Model file for the job. Use its own axes, mm. A direction names the side the tool comes from. Coordinates: 2 decimals unless noted, no trailing zeros. Loops run counter-clockwise (first coordinate to the right, second up) from the corner with the lowest first, then second, coordinate; pieces in that order, holes last.
from build123d import *

# Parameters (mm, degrees)
SKETCH_1_W          = 112
SKETCH_1_H          = 70
EXTRUDE_1_DEPTH     = 126
SKETCH_2_W          = 110
SKETCH_2_H          = 69
CUT_EXTRUDE_1_DEPTH = 125
SKETCH_3_W          = 112
SKETCH_3_H          = 1
EXTRUDE_2_DEPTH     = 12
SKETCH_4_W          = 22
SKETCH_4_H          = 1
EXTRUDE_3_DEPTH     = 12
CUT_EXTRUDE_2_DEPTH = 10
SKETCH_6_R          = 2.75
CUT_EXTRUDE_3_DEPTH = 190.770914526
CUT_EXTRUDE_5_REACH = 192.137
SKETCH_8_W          = 17
SKETCH_8_H          = 24
SKETCH_9_R          = 2.5
CUT_EXTRUDE_6_DEPTH = 10


with BuildPart() as part:
    # 草图1 → 拉伸1 (new body)
    with BuildSketch(Plane.XY):
        with Locations((56, 35)):
            Rectangle(SKETCH_1_W, SKETCH_1_H)
    extrude(amount=EXTRUDE_1_DEPTH)

    # 草图2 → 切除-拉伸1 (cut)
    with BuildSketch(Plane.XY.offset(126)):
        with Locations((56, 35.5)):
            Rectangle(SKETCH_2_W, SKETCH_2_H)
    extrude(amount=-CUT_EXTRUDE_1_DEPTH, mode=Mode.SUBTRACT)

    # 草图3 → 拉伸2 (add)
    with BuildSketch(Plane(origin=(0, 0, 0), x_dir=(-1, 0, 0), z_dir=(0, 0, -1))):
        with Locations((-56, 69.5)):
            Rectangle(SKETCH_3_W, SKETCH_3_H)
    extrude(amount=EXTRUDE_2_DEPTH)

    # 草图4 → 拉伸3 (add)
    with BuildSketch(Plane(origin=(112, 0, 0), x_dir=(0, 0, -1), z_dir=(1, 0, 0))):
        with Locations((-86, 69.5)):
            Rectangle(SKETCH_4_W, SKETCH_4_H)
    extrude_3 = extrude(amount=EXTRUDE_3_DEPTH)

    # 草图5 → 切除-拉伸2 (cut)
    with BuildSketch(Plane(origin=(0, 70, 0), x_dir=(-1, 0, 0), z_dir=(0, 1, 0))):
        Polygon((-112, 75), (-124, 87), (-124, 75), align=None)
    cut_extrude_2 = extrude(amount=-CUT_EXTRUDE_2_DEPTH, mode=Mode.SUBTRACT)

    # 镜向1: 拉伸3 across plane
    add(extrude_3.mirror(Plane.ZY.offset(-56)))

    # 镜向2: 切除-拉伸2 across plane
    add(cut_extrude_2.mirror(Plane.ZY.offset(-56)), mode=Mode.SUBTRACT)

    # 草图6 → 切除-拉伸3 (cut, through all)
    with BuildSketch(Plane.XZ.offset(-69)):
        with Locations(Location((-6, 90, 0), (0, 0, 270))):
            Circle(SKETCH_6_R)
        with Locations(Location((118, 90, 0), (0, 0, 270))):
            Circle(SKETCH_6_R)
        with Locations(Location((16, -6, 0), (0, 0, 270))):
            Circle(SKETCH_6_R)
        with Locations(Location((96, -6, 0), (0, 0, 270))):
            Circle(SKETCH_6_R)
    extrude(amount=-CUT_EXTRUDE_3_DEPTH, mode=Mode.SUBTRACT)

    # 草图8 → 切除-拉伸5 (cut, up to next)
    with BuildSketch(Plane.ZY, mode=Mode.PRIVATE) as cut_extrude_5_sk1:
        with Locations((117.5, 20)):
            Rectangle(SKETCH_8_W, SKETCH_8_H)
    cut_extrude_5_tool1 = extrude(cut_extrude_5_sk1.sketch, amount=-CUT_EXTRUDE_5_REACH, mode=Mode.PRIVATE) & part.part
    add(cut_extrude_5_tool1.solids().sort_by_distance((0, 20, 117.5))[0], mode=Mode.SUBTRACT)

    # 草图9 → 切除-拉伸6 (cut)
    with BuildSketch(Plane.ZY):
        with Locations((20, 65)):
            Circle(SKETCH_9_R)
        with Locations((20, 55)):
            Circle(SKETCH_9_R)
        with Locations((50, 65)):
            Circle(SKETCH_9_R)
        with Locations((50, 55)):
            Circle(SKETCH_9_R)
        with Locations((76, 25)):
            Circle(SKETCH_9_R)
        with Locations((76, 15)):
            Circle(SKETCH_9_R)
    extrude(amount=-CUT_EXTRUDE_6_DEPTH, mode=Mode.SUBTRACT)


solid = part.part
Q1. Flat gauge pins, fed straight in: P1, Ø12, axis at y = 13, z = 6.5, coming from the +X side; P2, Ø3.5, axis at x = 64, z = -7, coming from the -Y side; P3, Ø1.5, axis at x = 110, y = 31, coming from the -Z side. Where does each tip first touch, or does it go through?
Answers:
P1: stops at x = 112
P2: stops at y = 69
P3: stops at z = 0
Q2. Drill centre lines: line 1 (Y direction, x = 0.6, z = 76); line 2 (X direction, y = 20, z = 78); line 3 (Z direction, x = 61.5, y = 48.5). Where is each one in solid material? Low to high.
Answers:
line 1: y = 0 to 12.5, 17.5 to 22.5, 27.5 to 70
line 2: x = 0 to 1, 111 to 112
line 3: z = 0 to 1
Q3. Slice it at B-B (z = 50). List the corners of the cut face in (x, y), and give its area (3 significant figures).
Answers:
outline: (0, 0) - (112, 0) - (112, 70) - (111, 70) - (111, 1) - (1, 1) - (1, 52.5) - (0, 52.5) - close; (0, 57.5) - (1, 57.5) - (1, 62.5) - (0, 62.5) - close; (0, 67.5) - (1, 67.5) - (1, 70) - (0, 70) - close
area: 240 mm2
Q4. Which spindle directions (+Z, -Z, +X, -X, +Y, -Y) get a long thin tool onto all of the face, cutting with end or side? Do faces 1 (the cylindrical face through (116.327, 69.493, 92.182)), 2 (the flat face through (-3, 69, 89)), 3 (the flat face through (111, 35, 64)), 4 (the flat face through (55, 0, 62)), 5 (the cylindrical face through (0.49, 54.04, 52.31)). Say none if no direction does.
Answers:
face 1: +Y, -Y
face 2: +Z, -Z, -X, -Y
face 3: +Z, +Y
face 4: +Z, -Z, +X, -X, -Y
face 5: -X
Q5. Mould opens along X. For faces 6 (the flat face through (1, 35, 64)), 7 (the flat face through (115, 69, 89)) say: +X half, -X half, draft (parallel to the pull), parting line (faces both ways), or undercut.
Answers:
face 6: undercut
face 7: draft
Q6. Slice it at C-C (x = 96). List the corners of the cut face in (y, z), and give its area (4 significant figures).
Answers:
outline: (0, 0) - (69, 0) - (69, -3.25) - (70, -3.25) - (70, 1) - (1, 1) - (1, 126) - (0, 126) - close; (69, -12) - (70, -12) - (70, -8.75) - (69, -8.75) - close
area: 201.5 mm2
Q7. Slice it at D-D (y = 25). List the corners of the cut face in (x, z), and give its area (3 significant figures).
Answers:
outline: (0, 0) - (112, 0) - (112, 126) - (111, 126) - (111, 1) - (1, 1) - (1, 73.5) - (0, 73.5) - close; (0, 78.5) - (1, 78.5) - (1, 109) - (0, 109) - close
area: 340 mm2
Q8. Slice it at A-A (y = 65). List the corners of the cut face in (x, z).
Answers:
outline: (0, 0) - (112, 0) - (112, 126) - (111, 126) - (111, 1) - (1, 1) - (1, 17.5) - (0, 17.5) - close; (0, 22.5) - (1, 22.5) - (1, 47.5) - (0, 47.5) - close; (0, 52.5) - (1, 52.5) - (1, 126) - (0, 126) - close
